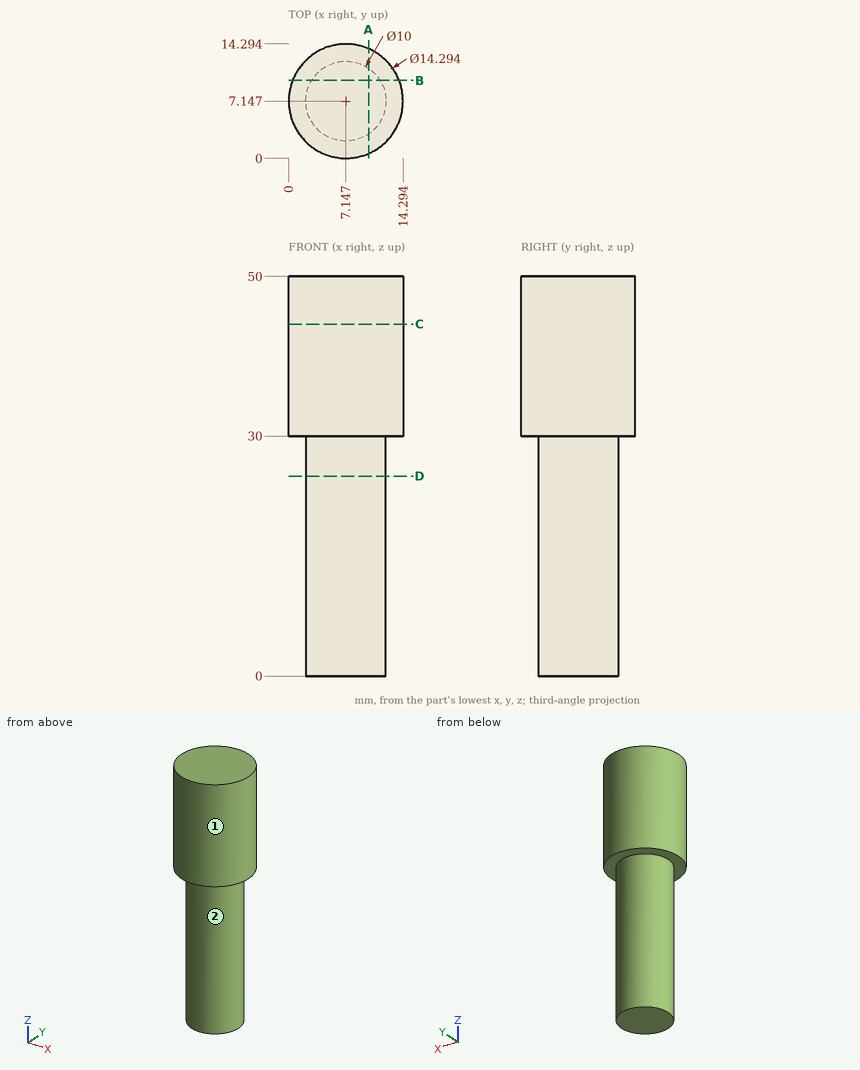
Source: three-view drawing plus pictorial views. Frame: mm from the lowest corner of the part. A direction names the side the tool comes from. Coordinates: 2 decimals unless noted, no trailing zeros. Loops run counter-clockwise (first coordinate to the right, second up) from the corner with the lowest first, then second, coordinate; pieces in that order, holes last. Notation, with made-up numbers: (-2.75, 10.25) - (45.25, 10.25) arc R21 ccw to (45.25, 20.25) - close; hole circle Ø4 at (32, 67.25). An arc over 180 degrees is marked (long way). Answer in a Markdown table with one row per item. Add a question column.
Item 1: Section query B-B on y = 9.75. Return the cut outline in (x, z) (1 decimal).
Item 2: Section query A-A on x = 10. Return the cut outline in (y, z) (1 decimal).
Item 3: Line query: line 1 along Z through (x, y) = (10.5, 3.25); line 2 along X through (y, z) = (10.5, 8) (1 decimal); line 3 along X through (y, z) = (10.25, 34) (1 decimal). Output: solid intervals per line, ascending. Write a range as [from, to].
Item 4: Section query D-D on z = 25. Return the cut outline in (x, y).
Item 5: Section query C-C on z = 44. Return the cut outline in (x, y).
Item 6: Contact query for flat-ended pins moving along their axis: P1, Ø5, axis at x = 9.5, z = 21.5, coming from the +Y side; P2, Ø1.5, axis at x = 12.5, z = 33, coming from the -Y side; P3, Ø5, axis at x = 7, z = 22.5, coming from the -Y side. Output: stop coordinate, or through.
Item 7: Access query for the marked faces 1 and 2. Directions: +Z, -Z, +X, -X, +Y, -Y. A direction counts if a zero-diameter tool reaches every point of the face in a straight line with its end or side. Return the directions, or none.
Recorded:
| question | item | result |
|---|---|---|
| 1 | outline | (0.5, 30) - (2.9, 30) - (2.9, 0) - (11.4, 0) - (11.4, 30) - (13.8, 30) - (13.8, 50) - (0.5, 50) - close |
| 2 | outline | (0.6, 30) - (3, 30) - (3, 0) - (11.3, 0) - (11.3, 30) - (13.7, 30) - (13.7, 50) - (0.6, 50) - close |
| 3 | line 1 | [30, 50] |
| 3 | line 2 | [3.4, 10.9] |
| 3 | line 3 | [0.7, 13.6] |
| 4 | outline | circle Ø10 at (7.15, 7.15) |
| 5 | outline | circle Ø14.29 at (7.15, 7.15) |
| 6 | P1 | y = 12.15 |
| 6 | P2 | y = 1.68 |
| 6 | P3 | y = 2.15 |
| 7 | face 1 | +Z, -Z |
| 7 | face 2 | -Z |
